Check sheet for the modelled part. Datum: model origin and axes. Units: mm. A direction names the side the tool comes from. Coordinates: 2 decimals unless noted, no trailing zeros. Loops run counter-clockwise (first coordinate to the right, second up) from the corner with the lowest first, then second, coordinate; pieces in that order, holes last.
```python
from build123d import *

# Parameters (mm, degrees)
F0_W      = 25.4
F0_H      = 25.4
F1_DEPTH  = 12.7
F1_FACE_W = 25.4
F1_FACE_H = 25.4
F2_DEPTH  = 12.7
F3_R      = 5.08
F7_R      = 2.308926
F7_R_2    = 2.30805
F7_R_3    = 2.2479
F7_R_4    = 2.311607
F7_R_5    = 2.312582
F7_R_6    = 2.312581
F10_DEPTH = 2.54
F6_R      = 6.538788
F11_DEPTH = 2.54
F4_R      = 2.2606
F12_DEPTH = 2.54
F5_R      = 3.8354
F13_DEPTH = 2.54
F8_R      = 2.3622
F14_DEPTH = 2.54
F9_R      = 2.9591
F15_DEPTH = 2.54


with BuildPart() as f1:
    # F0 (on Front) → F1 (new body)
    with BuildSketch(Plane.XZ):
        Rectangle(F0_W, F0_H)
    extrude(amount=F1_DEPTH)

    # F1_face (on face) → F2 (join)
    with BuildSketch(Plane(origin=(0, 0, 0), x_dir=(1, 0, 0), z_dir=(0, 1, 0))):
        Rectangle(F1_FACE_W, F1_FACE_H)
    extrude(amount=F2_DEPTH)

    # F3
    f3_edges = [f1.edges().sort_by_distance(p)[0] for p in [
        (0, -12.7, 12.7),
        (-12.7, -12.7, 0),
        (12.7, -12.7, 0),
        (12.7, 0, 12.7),
        (0, -12.7, -12.7),
        (-12.7, 0, -12.7),
        (12.7, 0, -12.7),
        (-12.7, 0, 12.7),
        (-12.7, 12.7, 0),
        (0, 12.7, -12.7),
        (12.7, 12.7, 0),
        (0, 12.7, 12.7),
    ]]
    fillet(f3_edges, radius=F3_R)

    # F7 (on face) → F10 (cut)
    with BuildSketch(Plane(origin=(0, 0, -12.7), x_dir=(1, 0, 0), z_dir=(0, 0, -1))):
        with Locations((-3.688791, -5.030171)):
            Circle(F7_R)
        with Locations((-3.569339, 0)):
            Circle(F7_R_2)
        with Locations((4.25537, -5.001526)):
            Circle(F7_R_3)
        with Locations((4.051426, 0)):
            Circle(F7_R_4)
        with Locations((3.942381, 4.969389)):
            Circle(F7_R_5)
        with Locations((-3.509941, 5.03017)):
            Circle(F7_R_6)
    extrude(amount=-F10_DEPTH, mode=Mode.SUBTRACT)

    # F6 (on face) → F11 (cut)
    with BuildSketch(Plane.XY.offset(12.7)):
        Circle(F6_R)
    extrude(amount=-F11_DEPTH, mode=Mode.SUBTRACT)

    # F4 (on face) → F12 (cut)
    with BuildSketch(Plane.XZ.offset(12.7)):
        Circle(F4_R)
        with Locations((-4.04017, 4.238222)):
            Circle(F4_R)
        with Locations((4.417736, 4.066108)):
            Circle(F4_R)
        with Locations((-4.146772, -3.964508)):
            Circle(F4_R)
        with Locations((3.975104, -3.964508)):
            Circle(F4_R)
    extrude(amount=-F12_DEPTH, mode=Mode.SUBTRACT)

    # F5 (on face) → F13 (cut)
    with BuildSketch(Plane(origin=(0, 12.7, 0), x_dir=(-1, 0, 0), z_dir=(0, 1, 0))):
        with Locations((3.08777, 3.088401)):
            Circle(F5_R)
        with Locations((-3.340728, -2.967977)):
            Circle(F5_R)
    extrude(amount=-F13_DEPTH, mode=Mode.SUBTRACT)

    # F8 (on face) → F14 (cut)
    with BuildSketch(Plane(origin=(-12.7, 0, 0), x_dir=(0, -1, 0), z_dir=(-1, 0, 0))):
        Circle(F8_R)
        with Locations((3.981089, 4.393674)):
            Circle(F8_R)
        with Locations((-4.135615, -3.990615)):
            Circle(F8_R)
    extrude(amount=-F14_DEPTH, mode=Mode.SUBTRACT)

    # F9 (on face) → F15 (cut)
    with BuildSketch(Plane.YZ.offset(12.7)):
        with Locations((-3.688771, 3.876482)):
            Circle(F9_R)
        with Locations((3.727126, 3.728518)):
            Circle(F9_R)
        with Locations((-3.824933, -3.732581)):
            Circle(F9_R)
        with Locations((3.978793, -3.627112)):
            Circle(F9_R)
    extrude(amount=-F15_DEPTH, mode=Mode.SUBTRACT)


solid = f1.part
```
1) Section check A-A on y = -11. Enter the section's corners in (x, z), plus the area to 3 significant figures.
Answer sheet:
outline: (-11.41, -7.62) arc R3.79 ccw to (-7.62, -11.41) - (7.62, -11.41) arc R3.79 ccw to (11.41, -7.62) - (11.41, 7.62) arc R3.79 ccw to (7.62, 11.41) - (-7.62, 11.41) arc R3.79 ccw to (-11.41, 7.62) - close; hole circle Ø4.52 at (-4.15, -3.96); hole circle Ø4.52 at (-4.04, 4.24); hole circle Ø4.52 at (0, 0); hole circle Ø4.52 at (3.98, -3.96); hole circle Ø4.52 at (4.42, 4.07)
area: 428 mm2
2) Section check B-B on y = 10.75. Enter the section's corners in (x, z).
Answer sheet:
outline: (-11.62, -7.62) arc R4 ccw to (-7.62, -11.62) - (7.62, -11.62) arc R4 ccw to (11.62, -7.62) - (11.62, 7.62) arc R4 ccw to (7.62, 11.62) - (-7.62, 11.62) arc R4 ccw to (-11.62, 7.62) - close; hole circle Ø7.67 at (-3.09, 3.09); hole circle Ø7.67 at (3.34, -2.97)
3) Section check D-D on x = 9. Enter the section's corners in (y, z), plus the area to 3 significant figures.
Answer sheet:
outline: (-12.51, -7.62) arc R4.89 ccw to (-7.62, -12.51) - (7.62, -12.51) arc R4.89 ccw to (12.51, -7.62) - (12.51, 7.62) arc R4.89 ccw to (7.62, 12.51) - (-7.62, 12.51) arc R4.89 ccw to (-12.51, 7.62) - close
area: 605 mm2
4) Mould release check, pull along Z, two halves, no side actions. Record for faces 1 (the cylindrical face through (0.107, 11.172, 11.251)), 2 (the cylindrical face through (3.93, -11.45, 1.86)), 3 (the cylindrical face through (6.4, 4.33, -11.45)): +Z half, -Z half, draft (parallel to the pull), parting line (faces both ways), or undercut.
Answer sheet:
face 1: +Z half
face 2: undercut
face 3: draft
5) Set-up check for faces 4 (the flat face through (-4, -10.16, -4)), 5 (the flat face through (-4, 0, -10.16)), 6 (the flat face through (-10.16, 4, -4)), 7 (the cylindrical face through (11.448, -1.002, -2.844)): record each of +Z, -Z, +X, -X, +Y, -Y from which the full face is reachable in a straight line by a thin tool's end or side.
Answer sheet:
face 4: -Y
face 5: -Z
face 6: -X
face 7: +X
6) Scan lines: line 1 (Y direction, x = -10.5, z = -2); line 2 (Z direction, x = 2.5, y = -10.75); line 3 (X direction, y = 2, z = -2.75). Record each from-to range of solid material in increasing order.
Answer sheet:
line 1: y = -11.8 to -1.26, 1.26 to 2.86, 5.41 to 11.8
line 2: z = -11.62 to -5.68, -2.25 to 2.87, 5.26 to 11.62
line 3: x = -12.7 to 10.16
7) Section check C-C on z = 0. Enter the section's corners in (x, y), plus the area to 3 significant figures.
Answer sheet:
outline: (-12.7, -7.62) arc R5.08 ccw to (-7.62, -12.7) - (-2.26, -12.7) - (-2.26, -10.16) - (2.26, -10.16) - (2.26, -12.7) - (7.62, -12.7) arc R5.08 ccw to (12.7, -7.62) - (12.7, 7.62) arc R5.08 ccw to (7.62, 12.7) - (5.77, 12.7) - (5.77, 10.16) - (0.91, 10.16) - (0.91, 12.7) - (-0.81, 12.7) - (-0.81, 10.16) - (-5.36, 10.16) - (-5.36, 12.7) - (-7.62, 12.7) arc R5.08 ccw to (-12.7, 7.62) - (-12.7, 2.36) - (-10.16, 2.36) - (-10.16, -2.36) - (-12.7, -2.36) - close
area: 576 mm2
8) Depth check by flat-ended pin: pin 1 (2.5 mm diameter, centred on x = -4.5, z = 4.5, fed in from -Y); pin 2 (4 mm diameter, centred on x = -2, z = 3.5, fed in from +Y); pin 3 (5.5 mm diameter, centred on x = -3.57, y = 0, fed in from +Z); pin 4 (10 mm diameter, centred on x = 7, z = 8.5, fed in from -Y). Enter the tip coordinate at first touch or a pass-through.
Answer sheet:
pin 1: stops at y = -10.16
pin 2: stops at y = 10.16
pin 3: stops at z = 10.16
pin 4: stops at y = -12.7
